Geometry: final body of the model. Coordinates: model frame, mm. A direction names the side the tool comes from. Coordinates: 2 decimals unless noted, no trailing zeros. Loops run counter-clockwise (first coordinate to the right, second up) from the corner with the lowest first, then second, coordinate; pieces in that order, holes last. Notation, with made-up numbers: (-38.75, 63) - (6.25, 63) arc R22 ccw to (6.25, 88) - close; hole circle Ø1 at (38.25, 17.25). An arc over 180 degrees is marked (long way). Return JSON: item names as keys, results as strings.
Autodesk Inventor part; units mm, degrees
ref_plane "YZ Plane" through (0, 0, 0) normal (1, 0, 0) x (0, 1, 0)
ref_plane "XZ Plane" through (0, 0, 0) normal (0, 1, 0) x (-1, 0, 0)
ref_plane "XY Plane" through (0, 0, 0) normal (0, 0, 1) x (1, 0, 0)
sketch "Skizze1" plane through (0, 0, 0) normal (1, 0, 0) x (0, 1, 0)
  line L0 (0, 0) -> (144, 0)
  line L1 (144, 0) -> (144, -68)
  line L2 (144, -68) -> (0, -68)
  line L3 (0, -68) -> (0, 0)
  dimension "d0" = 144
  dimension "d1" = 68
extrude "Extrusion1" add sketch "Skizze1" along normal blind 16
sketch "Skizze2" plane through (0, 0, 0) normal (0, 0, 1) x (1, 0, 0)
  line L0 (0, 0) -> (0, 144) construction
  line L1 (0, 72) -> (16, 72) construction
  line L2 (16, 144) -> (16, 0) construction
  line L3 (0, 144) -> (16, 144) construction
  line L4 (8, 144) -> (8, 0) construction
  line L5 (0, 144) -> (16, 144) construction
  line L6 (0, 0) -> (16, 0) construction
  line L7 (0, 144) -> (16, 144) construction
  line L8 (16, 144) -> (16, 0) construction
  line L9 (16, 0) -> (0, 0) construction
  line L10 (0, 0) -> (0, 144) construction
  line L11 (0, 112) -> (16, 112) construction
  line L12 (0, 32) -> (16, 32) construction
  point P0 (8, 112)
  point P1 (8, 72)
  point P2 (8, 32)
  dimension "d4" = 40
  dimension "d5" = 40
hole "Bohrung1" at (8, 112, 0) at (8, 72, 0) at (8, 32, 0) direction (0, 0, -1) diameter 2.5 depth 30 tip angle 118
sketch "Skizze3" plane through (0, 144, 0) normal (0, 1, 0) x (1, 0, 0)
  line L0 (0, 0) -> (16, 0)
  line L1 (16, 0) -> (16, 68)
  line L2 (16, 68) -> (0, 68)
  line L3 (0, 68) -> (0, 0)
  line L4 (8, 0) -> (8, 68) construction
  line L5 (0, 68) -> (16, 68) construction
  line L6 (16, 0) -> (16, 68) construction
  line L7 (16, 34) -> (0, 34) construction
  line L8 (0, 68) -> (0, 0) construction
  line L9 (0, 14) -> (16, 14) construction
  line L10 (0, 54) -> (16, 54) construction
  point P0 (8, 14)
  point P1 (8, 54)
  dimension "d13" = 14
  dimension "d22" = 14
hole "Bohrung2" at (8, 144, -14) at (8, 144, -54) direction (0, -1, 0) diameter 2.5 depth 25 tip angle 118
sketch "Skizze4" plane through (0, 0, -68) normal (0, 0, -1) x (-1, 0, 0)
  line L0 (0, 0) -> (-16, 0) construction
  line L1 (-16, 0) -> (-16, 144) construction
  line L2 (-16, 144) -> (0, 144) construction
  line L3 (0, 144) -> (0, 0) construction
  line L4 (-8, 0) -> (-8, 144) construction
  line L5 (-16, 144) -> (-16, 0) construction
  line L6 (-16, 72) -> (0, 72) construction
  circle A0 centre (-8, 72) radius 1.25 construction
  point P0 (-8, 112)
  point P1 (-8, 32)
  dimension "d23" = 40
  dimension "d24" = 40
hole "Bohrung3" at (8, 72, -68) at (8, 112, -68) at (8, 32, -68) direction (0, 0, 1) diameter 2.5 depth 30 tip angle 118
sketch "Skizze5" plane through (16, 0, 0) normal (1, 0, 0) x (0, 0, -1)
  line L0 (0, 0) -> (68, 0) construction
  line L1 (68, 0) -> (68, 144) construction
  line L2 (68, 144) -> (0, 144) construction
  line L3 (0, 144) -> (0, 0) construction
  line L4 (0, 0) -> (68, 0) construction
  line L5 (34, 0) -> (34, 144) construction
  line L6 (0, 72) -> (68, 72) construction
  line L7 (68, 73.25) -> (68, 70.75) construction
  point P0 (34, 52)
  point P1 (34, 92)
  dimension "d32" = 20
  dimension "d33" = 20
hole "Bohrung4" at (16, 52, -34) at (16, 92, -34) direction (-1, 0, 0) diameter 24 end through all
equation "\"d39\" = Stärke"
equation "\"Biegeradius\" = Stärke"
equation "\"BreiteBiegungsfreistellung\" = Stärke"
equation "\"TiefeBiegungsfreistellung\" = 0.5 * Stärke"
equation "\"GrößeEckenfreistellung\" = 4 * Stärke"
equation "\"MinimalRest\" = 2 * Stärke"
equation "\"Übergangsradius\" = Biegeradius"
equation "\"JacobiRadiusGröße\" = Biegeradius"
equation "\"Abstandsgröße\" = Stärke"
properties part number "licht_200_side_middle" material "Spanplatte"
Item 1: Section query C-C, the plane x = 4.25. Return loops of the section in (y, z).
Worked out:
{"outline": "(0, -68) - (144, -68) - (144, 0) - (0, 0) - close; hole circle Ø24 at (52, -34); hole circle Ø24 at (92, -34)"}
Item 2: Mould query, pull axis X, two halves, no side actions, for faces 5 (the face through (8.479, 113.155, -52.79)), 6 (the face through (16, 71, -34)), 7 (the face through (6, 71, 0)). Classes: +X half, -X half, draft (parallel to the pull), parting line (faces both ways), or undercut.
Worked out:
{"face 5": "undercut", "face 6": "+X half", "face 7": "draft"}
Item 3: Section query A-A, the plane y = 92. Return loops of the section in (x, z).
Worked out:
{"outline": "(0, -68) - (16, -68) - (16, -46) - (0, -46) - close; (0, -22) - (16, -22) - (16, 0) - (0, 0) - close"}
Item 4: First-contact query: pin 1 Ø21.5 at (y, z) = (52, -34) entering from -X; pin 2 Ø1.5 at (x, z) = (8, -54) entering from +Y; pin 3 Ø2 at (x, y) = (8, 32) entering from -Z; pin 4 Ø1.5 at (x, y) = (8, 112) entering from -Z. Flat tips, straight axial feed; report the tip coordinate or a pass-through.
Worked out:
{"pin 1": "through", "pin 2": "y = 118.7", "pin 3": "z = -37.85", "pin 4": "z = -37.7"}
Item 5: Section query D-D, the plane y = 49.5. Return loops of the section in (x, z), and give its area (3 significant figures).
Worked out:
{"outline": "(0, -68) - (16, -68) - (16, -45.74) - (0, -45.74) - close; (0, -22.26) - (16, -22.26) - (16, 0) - (0, 0) - close", "area": "712 mm^2"}
Item 6: Section query B-B, the plane z = -34. Return loops of the section in (x, y), and give its area (3 significant figures).
Worked out:
{"outline": "(0, 0) - (16, 0) - (16, 40) - (0, 40) - close; (0, 64) - (16, 64) - (16, 80) - (0, 80) - close; (0, 104) - (16, 104) - (16, 144) - (0, 144) - close", "area": "1,540 mm^2"}
Item 7: Reachability of faces 1 (the face through (7.62, 131.32, -52.81)), 2 (the face through (8.479, 70.845, -15.21)), 3 (the face through (8.479, 73.155, -52.79)), 4 (the face through (0, 71, -34)) from +Z, -Z, +X, -X, +Y, -Y: full face, straight path, thin tool, end or side. Return the list, or none.
Worked out:
{"face 1": "+Y", "face 2": "+Z", "face 3": "-Z", "face 4": "+Z, -Z, -X, +Y, -Y"}
Item 8: Ray query, probe 1 along Y at (x, z) = (6.5, -34); probe 2 along Z at (x, y) = (8, 137.25); probe 3 along Z at (x, y) = (4.5, 52). Return the intervals inside material, ascending. Write a range as from..to.
Worked out:
{"probe 1": "0..40, 64..80, 104..144", "probe 2": "-68..-55.25, -52.75..-15.25, -12.75..0", "probe 3": "-68..-46, -22..0"}
